```python
from build123d import *

# Parameters (mm, degrees)
SKETCH1_W           = 80
SKETCH1_H           = 40
BOSS_EXTRUDE1_DEPTH = 22
SKETCH2_R           = 19
CUT_EXTRUDE1_DEPTH  = 20
SKETCH3_R           = 17.999999941
CUT_EXTRUDE2_DEPTH  = 92.651513899
SKETCH4_R           = 2.5
BOSS_EXTRUDE2_DEPTH = 10


with BuildPart() as part:
    # Sketch1 → Boss-Extrude1 (new body)
    with BuildSketch(Plane(origin=(0, 0, 0), x_dir=(1, 0, 0), z_dir=(0, 1, 0))):
        with Locations((40, 20)):
            Rectangle(SKETCH1_W, SKETCH1_H)
    extrude(amount=BOSS_EXTRUDE1_DEPTH)

    # Sketch2 → Cut-Extrude1 (cut)
    with BuildSketch(Plane.XZ):
        with Locations(Location((20.07, -20, 0), (0, 0, 270))):
            Circle(SKETCH2_R)
        with Locations(Location((59.93, -20, 0), (0, 0, 270))):
            Circle(SKETCH2_R)
    extrude(amount=-CUT_EXTRUDE1_DEPTH, mode=Mode.SUBTRACT)

    # Sketch3 → Cut-Extrude2 (cut, through all)
    with BuildSketch(Plane.XZ.offset(-20)):
        with Locations(Location((20.07, -20, 0), (0, 0, 270))):
            Circle(SKETCH3_R)
        with Locations(Location((59.93, -20, 0), (0, 0, 270))):
            Circle(SKETCH3_R)
    extrude(amount=-CUT_EXTRUDE2_DEPTH, mode=Mode.SUBTRACT)

    # Sketch4 → Boss-Extrude2 (add)
    with BuildSketch(Plane(origin=(0, 22, 0), x_dir=(1, 0, 0), z_dir=(0, 1, 0))):
        with Locations(Location((4, 36, 0), (0, 0, 90))):
            Circle(SKETCH4_R)
        with Locations(Location((76, 36, 0), (0, 0, 90))):
            Circle(SKETCH4_R)
        with Locations(Location((76, 4, 0), (0, 0, 90))):
            Circle(SKETCH4_R)
        with Locations(Location((4, 4, 0), (0, 0, 90))):
            Circle(SKETCH4_R)
    extrude(amount=BOSS_EXTRUDE2_DEPTH)


solid = part.part
```
The model under review builds one solid part; all positions refer to its coordinate system, in mm. A direction names the side the tool comes from. Coordinates: 2 decimals unless noted, no trailing zeros. Write each loop counter-clockwise with the first axis right and the second up, starting at its lowest first coordinate (ties: lowest second). Pieces come first, ordered by that corner, then holes. Notation, with made-up numbers: (48, 76) - (103, 76) arc R18 ccw to (103, 83) - close; hole circle Ø8 at (30, 88). An arc over 180 degrees is marked (long way). Write item = value, one per line.
(1) Mouldability with a two-part tool opening along X and no side actions: class faces 4 (the face through (76, 32, -4)), 5 (the face through (25.477, 20.986, -37.169)), 6 (the face through (80, 11, -20)), 7 (the face through (0, 11, -20)) as pulls with the +X half, pulls with the -X half, needs draft (parallel to the pull), parting line crosses it, or undercut.
Result sheet:
face_4 = needs draft
face_5 = undercut
face_6 = pulls with the +X half
face_7 = pulls with the -X half
(2) Consider section D-D, the plane z = -20. Give the boundary of the cut face in (x, y).
Result sheet:
outline = (0, 0) - (1.07, 0) - (1.07, 20) - (2.07, 20) - (2.07, 22) - (0, 22) - close; (38.07, 20) - (39.07, 20) - (39.07, 0) - (40.93, 0) - (40.93, 20) - (41.93, 20) - (41.93, 22) - (38.07, 22) - close; (77.93, 20) - (78.93, 20) - (78.93, 0) - (80, 0) - (80, 22) - (77.93, 22) - close
(3) Consider section A-A, the plane x = 20.07. Give the boundary of the cut face in (y, z), then the cut area to 3 significant figures.
Result sheet:
outline = (0, -40) - (22, -40) - (22, -38) - (20, -38) - (20, -39) - (0, -39) - close; (0, -1) - (20, -1) - (20, -2) - (22, -2) - (22, 0) - (0, 0) - close
area = 48.0 mm^2
(4) Machinability: for faces 1 (the face through (12.79, 9.86, -37.55)), 2 (the face through (40, 22, -20)), 3 (the face through (40, 0, -19)), which of the approach directions +Z, -Z, +X, -X, +Y, -Y give a long, thin tool a straight path to every point of the face, cutting with its end or side? Answer none if there is none.
Result sheet:
face_1 = -Y
face_2 = +Y
face_3 = +Z, -Z, +X, -X, -Y
(5) Consider section B-B, the plane z = -11.5. Give the boundary of the cut face in (x, y).
Result sheet:
outline = (0, 0) - (3.08, 0) - (3.08, 20) - (4.2, 20) - (4.2, 22) - (0, 22) - close; (35.94, 20) - (37.06, 20) - (37.06, 0) - (42.94, 0) - (42.94, 20) - (44.06, 20) - (44.06, 22) - (35.94, 22) - close; (75.8, 20) - (76.92, 20) - (76.92, 0) - (80, 0) - (80, 22) - (75.8, 22) - close
(6) For P1, Ø1.5, axis at y = 20, z = -8, coming from the -X side; P2, Ø4, axis at x = 70, y = 24.5, coming from the +Z side, all flat-tipped, find the tip position at first contact; note any pin that passes through.
Result sheet:
P1 = 0
P2 = through
(7) For line 1 (X direction, y = 21.2, z = -20); line 2 (X direction, y = 14, z = -20); line 3 (Z direction, x = 59.5, y = 5), list the stretches that pass through material, from the lowest coordinate up. Write a range as [from, to].
Result sheet:
line_1 = [0, 2.07], [38.07, 41.93], [77.93, 80]
line_2 = [0, 1.07], [39.07, 40.93], [78.93, 80]
line_3 = [-40, -39], [-1, 0]
(8) Consider section C-C, the plane y = 12.5. Give the boundary of the cut face in (x, z).
Result sheet:
outline = (0, -40) - (80, -40) - (80, 0) - (0, 0) - close; hole circle Ø38 at (20.07, -20); hole circle Ø38 at (59.93, -20)
